Verification items for the finished model (mm, model axes). Face numbers are marked on the shaded views. A direction names the side the tool comes from. Round coordinates to 2 decimals unless told otherwise and drop trailing zeros. Order: outer loops, then holes, each group sorted by start corner. A loop starts at its lowest first (then second) coordinate and runs counter-clockwise, first axis right, second up. Notation, with made-up numbers: (-34, -24) -> (-1, -24) arc R10 cw to (-1, -18) -> close; hole circle Ø2 at (83.5, 73). An arc over 180 degrees is marked (long way). Return JSON: item names as keys, results as strings. Group by question number.
1) Depth check by flat-ended pin: pin 1 (1 mm diameter, centred on y = 122.5, z = -14.5, fed in from -X); pin 2 (2 mm diameter, centred on x = 227.5, z = 2, fed in from +Y). Enter the tip coordinate at first touch or a pass-through.
2) Section check B-B on y = 400. Enter the section's corners in (x, z), plus the area to 3 significant figures.
3) Scan lines: L1, parallel to Y at x = 300, z = -14; L2, parallel to Z at x = 343, y = 40; L3, parallel to Y at x = 286, z = -0.5. Record each from-to range of solid material in increasing order.
4) Section check C-C on x = 213.29. Enter the section's corners in (y, z) (3 decimals).
5) Section check A-A on x = 300. Enter the section's corners in (y, z).
6) Tool access check on the marked faces 1 and 2. Record the directions out of +Z, -Z, +X, -X, +Y, -Y that give a thin tool (end or side, any length) a straight path to the whole face; none if there is none.
7) Section check D-D on y = 28.5. Enter the section's corners in (x, z).
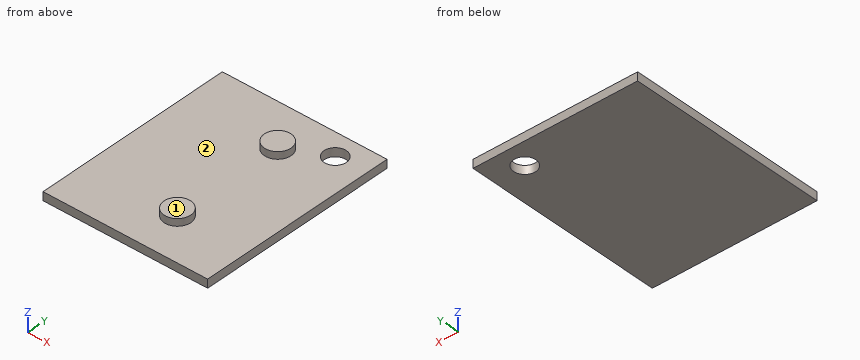
```python
from build123d import *

# Parameters (mm, degrees)
PAD_DEPTH    = 19
SKETCH002_R  = 25
POCKET_DEPTH = 19.001
SKETCH003_R  = 30
PAD001_DEPTH = 16


with BuildPart() as part:
    # Sketch → Pad (new body)
    with BuildSketch(Plane.XY):
        Polygon((0, 413.879036), (0, 452), (370, 452), (370, 0), (0, 0), align=None)
    extrude(amount=-PAD_DEPTH)

    # Sketch002 (on Face6 of Pad) → Pocket (cut, through all)
    with BuildSketch(Plane.XY):
        with Locations((300, 400)):
            Circle(SKETCH002_R)
    extrude(amount=-POCKET_DEPTH, mode=Mode.SUBTRACT)

    # Sketch003 (on Face4 of Pocket) → Pad001 (join)
    with BuildSketch(Plane.XY):
        with Locations((213.29, 352.375)):
            Circle(SKETCH003_R)
        with Locations((213.29, 99.625)):
            Circle(SKETCH003_R)
    extrude(amount=PAD001_DEPTH)


solid = part.part
```
Check result:
{
 "1": {"pin 1": "x = 0", "pin 2": "y = 379.31"},
 "2": {"outline": "(0, -19) -> (275, -19) -> (275, 0) -> (0, 0) -> close; (325, -19) -> (370, -19) -> (370, 0) -> (325, 0) -> close", "area": "6,080 mm^2"},
 "3": {"L1": "0 to 375, 425 to 452", "L2": "-19 to 0", "L3": "0 to 379.29, 420.71 to 452"},
 "4": {"outline": "(0, -19) -> (452, -19) -> (452, 0) -> (382.375, 0) -> (382.375, 16) -> (322.375, 16) -> (322.375, 0) -> (129.625, 0) -> (129.625, 16) -> (69.625, 16) -> (69.625, 0) -> (0, 0) -> close"},
 "5": {"outline": "(0, -19) -> (375, -19) -> (375, 0) -> (0, 0) -> close; (425, -19) -> (452, -19) -> (452, 0) -> (425, 0) -> close"},
 "6": {"face 1": "+Z, +X, -X, +Y, -Y", "face 2": "+Z"},
 "7": {"outline": "(0, -19) -> (370, -19) -> (370, 0) -> (0, 0) -> close"}
}
